Part model, mm, in its own coordinate system. A direction names the side the tool comes from. Round coordinates to 2 decimals unless told otherwise and drop trailing zeros. Loops run counter-clockwise (first coordinate to the right, second up) from the corner with the lowest first, then second, coordinate; pieces in that order, holes last. Notation, with made-up numbers: (62.25, -23) -> (94.25, -23) arc R18 cw to (94.25, -5) -> close; hole circle Ø10 at (69.5, 27.25). An arc over 180 degrees is marked (long way). Answer as CSV lines item,"result".
from build123d import *

# Parameters (mm, degrees)
SKETCH1_R           = 10.325
BOSS_EXTRUDE1_DEPTH = 32.9438
SKETCH2_W           = 23.0124
SKETCH2_H           = 19.05
BOSS_EXTRUDE2_DEPTH = 1.5875


with BuildPart() as part:
    # Sketch1 → Boss-Extrude1 (new, symmetric)
    with BuildSketch(Plane.XY):
        Circle(SKETCH1_R)
    extrude(amount=BOSS_EXTRUDE1_DEPTH, both=True)

    # Sketch2 → Boss-Extrude2 (add, symmetric)
    # profile 1 of 2: a face of its own
    with BuildSketch(Plane(origin=(0, 0, 0), x_dir=(0, 0, -1), z_dir=(1, 0, 0))):
        with Locations((-44.45, 0)):
            Rectangle(SKETCH2_W, SKETCH2_H)
        with BuildLine():
            Line((-45.2501, 4.3688), (-46.0375, 4.3688))
            ThreePointArc((-46.0375, 4.3688), (-50.4063, 0), (-46.0375, -4.3688))
            Line((-46.0375, -4.3688), (-45.2501, -4.3688))
            ThreePointArc((-45.2501, -4.3688), (-40.8813, 0), (-45.2501, 4.3688))
        make_face(mode=Mode.SUBTRACT)
    # profile 2 of 2: a face of its own
    with BuildSketch(Plane(origin=(0, 0, 0), x_dir=(0, 0, -1), z_dir=(1, 0, 0))):
        with Locations((44.45, 0)):
            Rectangle(SKETCH2_W, SKETCH2_H)
        with BuildLine():
            Line((45.2501, -4.3688), (46.0375, -4.3688))
            ThreePointArc((46.0375, -4.3688), (50.4063, 0), (46.0375, 4.3688))
            Line((46.0375, 4.3688), (45.2501, 4.3688))
            ThreePointArc((45.2501, 4.3688), (40.8813, 0), (45.2501, -4.3688))
        make_face(mode=Mode.SUBTRACT)
    extrude(amount=BOSS_EXTRUDE2_DEPTH, both=True)


solid = part.part
Q1. Saw through at A-A, the plane x = 0. Write the cut outline in (y, z) (1 decimal), then the cut area to 3 significant figures.
Geometry results:
outline,"(-10.3, -32.9) -> (-9.5, -32.9) -> (-9.5, -56) -> (9.5, -56) -> (9.5, -32.9) -> (10.3, -32.9) -> (10.3, 32.9) -> (9.5, 32.9) -> (9.5, 56) -> (-9.5, 56) -> (-9.5, 32.9) -> (-10.3, 32.9) -> close; hole (-4.4, -46) arc R4.4 ccw to (4.4, -46) -> (4.4, -45.3) arc R4.4 ccw to (-4.4, -45.3) -> close; hole (-4.4, 45.3) arc R4.4 ccw to (4.4, 45.3) -> (4.4, 46) arc R4.4 ccw to (-4.4, 46) -> close"
area,"2,100 mm2"
Q2. Which spindle directions (+Z, -Z, +X, -X, +Y, -Y) get a long thin tool onto all of the face, cutting with end or side? Do faces 1 (the face through (0, -9.525, 45)), 2 (the face through (-1.588, 4, -42)), 3 (the face through (0.022, -0.096, -50.405)), 4 (the face through (-1.588, 4, 42)). Say none if no direction does.
Geometry results:
face 1,"+Z, +X, -X, -Y"
face 2,"-Z, -X, +Y, -Y"
face 3,"+X, -X"
face 4,"+Z, -X, +Y, -Y"
Q3. Saw through at B-B, the plane y = 0. Write the cut outline in (x, z) (1 decimal), then the cut area to 3 significant figures.
Geometry results:
outline,"(-10.3, -32.9) -> (-1.6, -32.9) -> (-1.6, -40.9) -> (1.6, -40.9) -> (1.6, -32.9) -> (10.3, -32.9) -> (10.3, 32.9) -> (1.6, 32.9) -> (1.6, 40.9) -> (-1.6, 40.9) -> (-1.6, 32.9) -> (-10.3, 32.9) -> close; (-1.6, -56) -> (1.6, -56) -> (1.6, -50.4) -> (-1.6, -50.4) -> close; (-1.6, 50.4) -> (1.6, 50.4) -> (1.6, 56) -> (-1.6, 56) -> close"
area,"1,450 mm2"
Q4. Saw through at C-C, the plane y = 7. Write the cut outline in (x, z), then the cut area to 3 significant figures.
Geometry results:
outline,"(-7.59, -32.94) -> (-1.59, -32.94) -> (-1.59, -55.96) -> (1.59, -55.96) -> (1.59, -32.94) -> (7.59, -32.94) -> (7.59, 32.94) -> (1.59, 32.94) -> (1.59, 55.96) -> (-1.59, 55.96) -> (-1.59, 32.94) -> (-7.59, 32.94) -> close"
area,"1,150 mm2"
Q5. Drop flat-ended pins along their axis: P1, Ø1.6, axis at x = -0.5, z = 45.5, coming from the +Y side (3 decimals); P2, Ø5.5, axis at y = -1, z = -48.5, coming from the +X side; P3, Ø6, axis at y = -4, z = 22.5, coming from the +X side. Give the stop position or say it passes through.
Geometry results:
P1,"y = 9.525"
P2,"x = 1.59"
P3,"x = 10.28"
Q6. Two-plate mould, pull along Z, no slides. Class faces 5 (the face through (0.022, 0.096, -40.882)), 6 (the face through (1.588, 4, -42)), 7 (the face through (0, 0, 55.956)): pulls with the +Z half, pulls with the -Z half, needs draft (parallel to the pull), parting line crosses it, or undercut.
Geometry results:
face 5,"undercut"
face 6,"needs draft"
face 7,"pulls with the +Z half"
Q7. Drill centre lines: line 1 along Z through (x, y) = (-0.25, -0.5); line 2 along Z through (x, y) = (5.25, -2.5); line 3 along X through (y, z) = (8.5, 50). Where is each one in solid material? Low to high.
Geometry results:
line 1,"-55.96 to -50.38, -40.91 to 40.91, 50.38 to 55.96"
line 2,"-32.94 to 32.94"
line 3,"-1.59 to 1.59"
Q8. Saw through at D-D, the plane z = -21. Write the cut outline in (x, y) (3 decimals), then the cut area to 3 significant figures.
Geometry results:
outline,"circle Ø20.65 at (0, 0)"
area,"335 mm2"
